Verification items for the finished model (mm, model axes). Face numbers are marked on the shaded views. A direction names the side the tool comes from. Coordinates: 2 decimals unless noted, no trailing zeros. Write each loop counter-clockwise with the first axis right and the second up, starting at its lowest first coordinate (ties: lowest second). Pieces come first, ordered by that corner, then holes. Notation, with made-up numbers: (-39.5, 46) -> (-6.5, 46) arc R14 ccw to (-6.5, 63) -> close; hole circle Ø9 at (69, -31). An arc over 180 degrees is marked (long way). Answer in a Markdown table with one row per item.
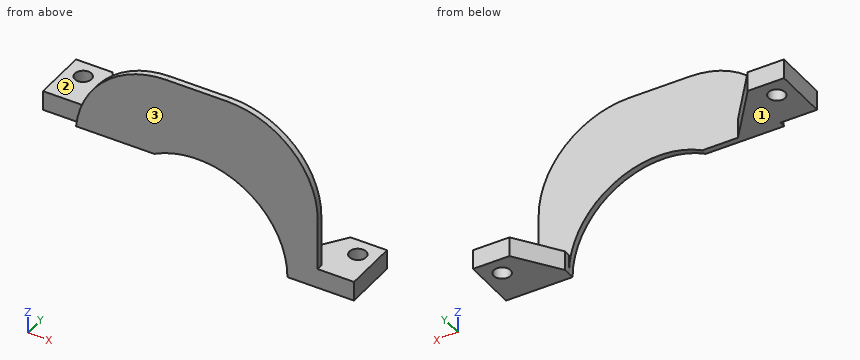
Autodesk Inventor part; units mm, degrees
ref_plane "YZ Plane" through (0, 0, 0) normal (1, 0, 0) x (0, 1, 0)
ref_plane "XZ Plane" through (0, 0, 0) normal (0, 1, 0) x (-1, 0, 0)
ref_plane "XY Plane" through (0, 0, 0) normal (0, 0, 1) x (1, 0, 0)
sketch "スケッチ1" plane through (0, 0, 0) normal (0, 1, 0) x (-1, 0, 0)
  line L0 (0, 0) -> (40, 0)
  line L1 (40, 0) -> (40, -26.8558)
  line L2 (40, -26.8558) -> (0, -26.8558)
  line L3 (0, -26.8558) -> (0, 0)
  circle A0 centre (20, -26.8558) radius 15
  line L4 (20, -26.8558) -> (20, 0)
  line L5 (40, -23.6058) -> (40, -26.8558)
  line L6 (0, -23.6058) -> (0, -26.8558)
  circle A1 centre (20, -26.8558) radius 17
  line L7 (40, -26.8558) -> (46, -26.8558)
  line L8 (46, -26.8558) -> (46, -23.6058)
  line L9 (46, -23.6058) -> (40, -23.6058)
  line L10 (40, -23.6058) -> (40, -26.8558)
  line L11 (0, -23.6058) -> (0, -26.8558)
  line L12 (0, -26.8558) -> (-6, -26.8558)
  line L13 (-6, -26.8558) -> (-6, -23.6058)
  line L14 (-6, -23.6058) -> (0, -23.6058)
  line L15 (0, -23.6058) -> (0, -26.8558)
  point P0 (35, -26.8558)
  point P1 (5, -26.8558)
  dimension "d0" = 40
  dimension "d1" = 30
  dimension "d16" = 34
  dimension "d18" = 6
  dimension "d19" = 3.25
extrude "押し出し1" add sketch "スケッチ1" along normal blind 1 contours L0 L4 A1 L2 L3 | L0 L1 L2 A1 L4 | A1 L2 A0 L4 | L4 A0 L2 A1 | L4 L2 A0 | A0 L2 L4
fillet "フィレット1" radius 15 2 edges at (-40, 0.5, 0) (0, 0.5, 0)
extrude "押し出し4" add sketch "スケッチ1" along normal blind 9 contours L3 L12 L13 L14 | L9 L8 L7 L1
sketch "スケッチ7" plane through (6, 0, -26.8558) normal (0, 0, -1) x (-1, 0, 0)
  circle A0 centre (3, 6) radius 1.375
  line L0 (6, 1) -> (6, 9)
  line L1 (0, 9) -> (6, 9)
  circle A1 centre (49.4019, 6) radius 1.375
  line L2 (46, 9) -> (52, 9)
  line L3 (52, 0) -> (52, 9)
  point P0 (6, 0)
  point P1 (3, 9)
  point P2 (52, 4.5)
  dimension "d22" = 2.75
  dimension "d23" = 3
  dimension "d24" = 3
  dimension "d25" = 2.75
  dimension "d26" = 3
  dimension "d27" = 3
extrude "押し出し5" cut sketch "スケッチ7" against normal blind 6
extrude "押し出し6" cut sketch "スケッチ1" along normal blind 1 contours L4 L2 A0 | A0 L2 L4
sketch "スケッチ9" plane through (6, 9, -26.8558) normal (0, 0, -1) x (-1, 0, 0)
  line L0 (6, -8) -> (6, 0)
  line L1 (6, -8) -> (11, -8)
  line L2 (11, -8) -> (11, -7)
  line L3 (11, -7) -> (6, -7)
  line L4 (6, -7) -> (6, -8)
  line L5 (6, 0) -> (11, -7)
  line L6 (41, -8) -> (41, -9)
  line L7 (52, 0) -> (46, 0)
  line L8 (46, -8) -> (46, 0)
  line L9 (46, -8) -> (41, -8)
  line L10 (41, -8) -> (41, -7)
  line L11 (41, -7) -> (46, -7)
  line L12 (46, -7) -> (46, -8)
  line L13 (46, 0) -> (41, -7)
  point P0 (6, -9)
  dimension "d32" = 5
  dimension "d33" = 1
  dimension "d38" = 5
extrude "押し出し7" add sketch "スケッチ9" against normal blind 3.25
sketch "スケッチ10" plane through (0, 1, 0) normal (0, 1, 0) x (1, 0, 0)
  line L0 (-35, 23.6058) -> (-40, 23.6058)
  line L1 (-40, 23.6058) -> (-35, 23.6058)
  line L2 (-35, 23.6058) -> (-35, 13.6058)
  line L3 (-35, 13.6058) -> (-40, 13.6058)
  line L4 (-40, 13.6058) -> (-40, 23.6058)
  line L5 (-40, 13.6058) -> (-27, 13.6058)
  line L6 (-27, 13.6058) -> (-27, 10.3558)
  line L7 (-27, 10.3558) -> (-40, 10.3558)
  line L8 (-40, 10.3558) -> (-40, 13.6058)
  line L9 (-24.5918, 17.2551) -> (-23.5955, 17.2551)
  line L10 (-23.5955, 17.2551) -> (-23.5955, 14.4656)
  line L11 (-23.5955, 14.4656) -> (-24.5918, 14.4656)
  line L12 (-24.5918, 14.4656) -> (-24.5918, 17.2551)
  arc A0 (-40, 15) -> (-25, 0) centre (-25, 15) ccw
  arc A1 (-40, 15) -> (-39.2629, 10.3558) centre (-25, 15) ccw
  line L13 (-40, 13.6058) -> (-46, 13.6058)
  line L14 (-46, 13.6058) -> (-46, 10.3558)
  line L15 (-46, 10.3558) -> (-40, 10.3558)
  line L16 (-40, 10.3558) -> (-40, 13.6058)
  point P0 (0, 0)
  dimension "d39" = 5
  dimension "d40" = 10
  dimension "d41" = 13
  dimension "d42" = 3.25
  dimension "d43" = 6
sketch "スケッチ11" plane through (-46, 0, -23.6058) normal (0, 0, 1) x (1, 0, 0)
  line L0 (0, 9) -> (6, 9)
  line L1 (6, 1) -> (6, 0)
  line L2 (6, 9) -> (6, 1)
  point P0 (46, 0)
extrude "押し出し8" add sketch "スケッチ10" along normal blind 9 contours L8 L15 L14 L13
sketch "スケッチ12" plane through (-46, 1, -10.3558) normal (0, 0, 1) x (1, 0, 0)
  line L0 (0, 0) -> (6, 0)
  line L1 (6, 0) -> (13.0551, 0)
  line L2 (0, 9) -> (6, 9)
  line L3 (13.0551, 0) -> (6, 9)
  line L4 (6, 0) -> (6, 9)
  line L5 (6, 0) -> (6, 9)
  point P0 (46, -1)
extrude "押し出し9" add sketch "スケッチ12" against normal blind 3.25
sketch "スケッチ13" plane through (-46, 1, -10.3558) normal (0, 0, 1) x (1, 0, 0)
  circle A0 centre (3, 6) radius 1.375
  line L0 (0, 9) -> (6, 9)
  line L1 (0, 0) -> (0, 9)
  point P0 (46, -1)
  dimension "d48" = 2.75
  dimension "d49" = 3
  dimension "d50" = 3
extrude "押し出し10" cut sketch "スケッチ13" against normal blind 3.25
sketch "スケッチ14" plane through (-46, 0, -23.6058) normal (0, 0, 1) x (1, 0, 0)
  line L0 (11, 1) -> (11, 2)
  line L1 (0, 9) -> (6, 9)
  line L2 (11, 1) -> (0, 1)
  line L3 (0, 1) -> (0, 9)
  line L4 (0, 9) -> (11, 9)
  line L5 (11, 9) -> (11, 1)
  line L6 (0, 1) -> (6, 1)
  line L7 (6, 1) -> (6, 0)
  line L8 (6, 0) -> (0, 0)
  line L9 (0, 0) -> (0, 1)
  point P0 (46, 0)
extrude "押し出し11" cut sketch "スケッチ14" against normal blind 9
sketch "スケッチ15" plane through (0, 1, 0) normal (0, 1, 0) x (1, 0, 0)
  arc A0 (-40, 15) -> (-39.9351, 13.6058) centre (-25, 15) ccw
  line L0 (-39.9351, 13.6058) -> (-27.0312, 13.6058)
  arc A1 (-35, 26.8558) -> (-5, 26.8558) centre (-20, 26.8558) ccw
  line L1 (-39.9351, 13.6058) -> (-32.9449, 13.6058)
  line L2 (-40, 26.8558) -> (-40, 15)
  line L3 (-39.9351, 13.6058) -> (-40, 26.8558)
  line L4 (-40, 26.8558) -> (-35, 26.8558)
  line L5 (-40, 26.8558) -> (-35, 26.8558)
  line L6 (-35, 26.8558) -> (-27.0312, 13.6058)
  arc A2 (-39.9351, 13.6058) -> (-39.2629, 10.3558) centre (-25, 15) ccw
  arc A3 (-40, 26.8558) -> (-39.9351, 13.6058) centre (466.0679, 22.7107) ccw
  point P0 (0, 0)
  point P1 (-40, 18.5657)
extrude "押し出し12" cut sketch "スケッチ15" against normal blind 9 contours L3 L4 A1 L0 | A3 L2 L3
sketch "スケッチ16" plane through (0, 1, 0) normal (0, 1, 0) x (1, 0, 0)
  arc A0 (-40, 15) -> (-39.9351, 13.6058) centre (-25, 15) ccw
  line L0 (-40, 18.5657) -> (-40, 15)
  line L1 (-39.9351, 13.6058) -> (-40, 18.5657)
  arc A1 (-40, 18.5657) -> (-39.9351, 13.6058) centre (0.7021, 16.6182) ccw
  point P0 (0, 0)
extrude "押し出し13" cut sketch "スケッチ16" against normal blind 9 contours L0 L1 A1 A0 | A0 A1 L0
sketch "スケッチ17" plane through (0, 1, 0) normal (0, 1, 0) x (1, 0, 0)
  arc A0 (-39.992, 14.51) -> (-39.9351, 13.6058) centre (-25, 15) ccw
  line L0 (-39.9351, 13.6058) -> (-27.0312, 13.6058)
  line L1 (-39.992, 14.51) -> (-39.9351, 14.51)
  line L2 (-39.9351, 14.51) -> (-39.9351, 13.6058)
  line L3 (-39.9351, 13.6058) -> (-39.992, 13.6058)
  line L4 (-39.992, 13.6058) -> (-39.992, 14.51)
  point P0 (0, 0)
extrude "押し出し14" cut sketch "スケッチ17" against normal blind 9
properties part number "PartsForRaspibase"
1. Thickness scan on line 1 (Y direction, x = 3, z = -25.9) (3 decimals); line 2 (Y direction, x = -43, z = -11.4) (3 decimals); line 3 (Y direction, x = -15, z = -7). Record the ranges inside material, lowest first. Write a range as from..to.
Geometry says:
| item | result |
|---|---|
| line 1 | 0..4.625, 7.375..9 |
| line 2 | 1..5.625, 8.375..10 |
| line 3 | 0..1 |
2. Section check C-C, the plane z = -9.5. Record the boundary of the cut face in (x, y).
Geometry says:
| item | result |
|---|---|
| outline | (-38.96, 0) -> (-1.04, 0) -> (-1.04, 1) -> (-38.96, 1) -> close |
3. Tool access check on the marked faces 1, 2 and 3. Record the directions out of +Z, -Z, +X, -X, +Y, -Y that give a thin tool (end or side, any length) a straight path to the whole face; none if there is none.
Geometry says:
| item | result |
|---|---|
| face 1 | -Z, -X, +Y, -Y |
| face 2 | +Z, +X, -X, +Y |
| face 3 | +Z, -Z, +X, -X, -Y |
4. Section check B-B, the plane x = 3. Record the boundary of the cut face in (y, z) (3 decimals).
Geometry says:
| item | result |
|---|---|
| outline | (0, -26.856) -> (4.625, -26.856) -> (4.625, -23.606) -> (0, -23.606) -> close; (7.375, -26.856) -> (9, -26.856) -> (9, -23.606) -> (7.375, -23.606) -> close |
5. Section check D-D, the plane x = -13. Record the boundary of the cut face in (y, z), plus the area to 3 significant figures.
Geometry says:
| item | result |
|---|---|
| outline | (0, -13.59) -> (1, -13.59) -> (1, -0.13) -> (0, -0.13) -> close |
| area | 13.5 mm^2 |
6. Section check A-A, the plane x = -43. Record the boundary of the cut face in (y, z) (3 decimals).
Geometry says:
| item | result |
|---|---|
| outline | (1, -13.606) -> (5.625, -13.606) -> (5.625, -10.356) -> (1, -10.356) -> close; (8.375, -13.606) -> (10, -13.606) -> (10, -10.356) -> (8.375, -10.356) -> close |
7. Depth check by flat-ended pin: P1, Ø3.5, axis at x = -44, z = -12, coming from the -Y side; P2, Ø1.1, axis at y = 1.5, z = -26, coming from the -X side; P3, Ø1.5, axis at y = 5.5, z = -12.5, coming from the +X side. Enter the tip coordinate at first touch or a pass-through.
Geometry says:
| item | result |
|---|---|
| P1 | y = 1 |
| P2 | x = -5.04 |
| P3 | x = -35.88 |
